Can you work these out from the model? Positions are in its coordinate system, mm. Face numbers are marked on the shaded views. A direction names the side the tool comes from. Give positions to 0.01 mm unless a question says otherwise; leave off trailing zeros. Order: outer loops, then holes, each group sorted by start corner. A loop starts at its lowest first (then second) coordinate and runs counter-clockwise, first axis right, second up. Notation, with made-up numbers: (3, -34) - (50, -34) arc R18 ccw to (50, -25) - close; hole circle Ø1 at (67, 73). An arc over 180 degrees is marked (long way). Return JSON: item names as keys, results as strings.
```python
from build123d import *

# Parameters (mm, degrees)
F1_DEPTH = 63.5
F0_W     = 25.4
F0_H     = 17.965186498
F2_DEPTH = 25.4
F3_DEPTH = 7.9375
F5_R     = 6.35


with BuildPart() as f1:
    # F0 (on Front) → F1 (new body, symmetric)
    with BuildSketch(Plane.XZ):
        Polygon((38.8800390695, 20.1806084275), (-24.6199609305, 20.1806084275), (-24.6199609305, 1.1306084275), (57.9300390695, 1.1306084275), (57.9300390695, 20.1806084275), align=None)
    extrude(amount=F1_DEPTH, both=True)

    # F0 (on Front) → F2 (join, symmetric)
    with BuildSketch(Plane.XZ):
        with Locations((91.4859331562, 62.5134016765)):
            Rectangle(F0_W, F0_H)
        with BuildLine():
            Line((38.8800390695, 36.0163077712), (38.8800390695, 20.1806084275))
            Line((38.8800390695, 20.1806084275), (57.9300390695, 20.1806084275))
            Line((57.9300390695, 20.1806084275), (57.9300390695, 36.5266351785))
            ThreePointArc((57.9300390695, 36.5266351785), (62.4384600836, 48.0819539272), (73.5812261701, 53.5308084275))
            Line((73.5812261701, 53.5308084275), (78.7859331562, 53.5308084275))
            Line((78.7859331562, 53.5308084275), (78.7859331562, 71.4959949255))
            Line((78.7859331562, 71.4959949255), (73.5812261701, 71.4959949255))
            add(Edge.make_bspline(
                [(73.0621663059, 71.4806777175), (73.2353354158, 71.485987393), (73.4083566499, 71.4910929714), (73.5812261701, 71.4959949255)],
                knots=[110.3659801148, 110.3659801148, 110.3659801148, 110.3659801148, 110.8004604656, 110.8004604656, 110.8004604656, 110.8004604656], degree=3))
            ThreePointArc((73.0621663059, 71.4806777175), (48.816685952, 60.6442358108), (38.8800390695, 36.0163077712))
        make_face()
    extrude(amount=F2_DEPTH, both=True)

    # F0 (on Front) → F3 (join, symmetric)
    with BuildSketch(Plane.XZ):
        with BuildLine():
            add(Edge.make_bspline(
                [(-24.6199609305, 20.1806084275), (-24.4558339647, 55.6137443141), (29.0740353989, 70.1319227371), (73.0621663059, 71.4806777175)],
                knots=[0, 0, 0, 0, 110.3659801148, 110.3659801148, 110.3659801148, 110.3659801148], degree=3))
            Line((-24.6199609305, 20.1806084275), (38.8800390695, 20.1806084275))
            Line((38.8800390695, 20.1806084275), (38.8800390695, 36.0163077712))
            ThreePointArc((38.8800390695, 36.0163077712), (48.816685952, 60.6442358108), (73.0621663059, 71.4806777175))
        make_face()
    extrude(amount=F3_DEPTH, both=True)

    # F0 (on Front) → F4 (revolve)
    with BuildSketch(Plane.XZ):
        Polygon((104.1859331562, 77.3306084275), (104.1859331562, 71.4959949255), (104.1859331562, 53.5308084275), (104.1859331562, 48.7556084275), (129.5859331562, 48.7556084275), (129.5859331562, 77.3306084275), align=None)
    revolve(axis=Axis((104.1859331562, 0, 63.0431084275), (0, 0, -1)))

    # F5
    f5_edges = [f1.edges().sort_by_distance(p)[0] for p in [
        (57.930039, 63.5, 10.655608),
        (57.930039, -63.5, 10.655608),
        (-24.619961, 63.5, 10.655608),
        (-24.619961, -63.5, 10.655608),
    ]]
    fillet(f5_edges, radius=F5_R)


solid = f1.part
```
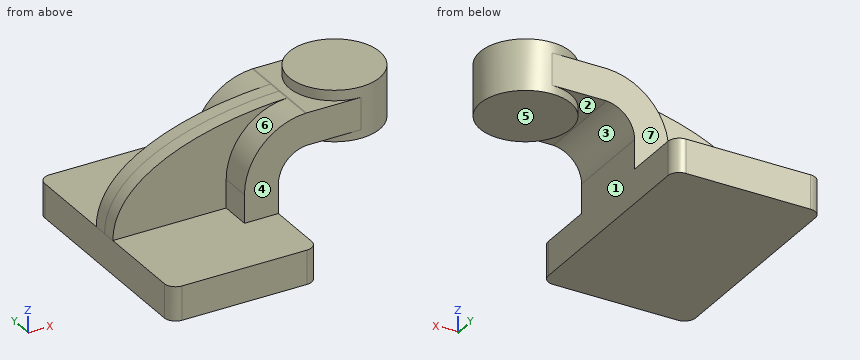
1. Thinking about a two-plate mould opening in X: for the marked faces 1, 2, 3 and 4, which applies, +X half, -X half, draft (parallel to the pull), parting line (faces both ways), or undercut?
Checks:
{"face 1": "+X half", "face 2": "undercut", "face 3": "undercut", "face 4": "draft"}
2. On a 3-axis mill with a long thin cutter (end or side, diameter ignored), from which of +Z, -Z, +X, -X, +Y, -Y can I reach the whole of each face in a straight line? I mean the marked faces 5, 6 and 7. Say none if no direction works.
Checks:
{"face 5": "-Z, +X, +Y, -Y", "face 6": "+Z, -X, -Y", "face 7": "+Z, +X, -X, +Y"}
3. If I drill on L1, parallel to Z at x = 32, y = 48; L2, parallel to Z at x = 86, y = -21; L3, parallel to X at y = -52.5, z = 8, over which ranges is the centre line in solid material (lowest first)? Write a range as [from, to].
Checks:
{"L1": "[1.13, 20.18]", "L2": "[53.53, 71.5]", "L3": "[-24.62, 57.93]"}
4. Suppose I cut it at B-B (y = -44). List the corners of the cut face in (x, z) for me.
Checks:
{"outline": "(-24.62, 1.13) - (57.93, 1.13) - (57.93, 20.18) - (-24.62, 20.18) - close"}
5. For pin 1 Ø16.5 at (x, y) = (5.5, -24) entering from +Z; pin 2 Ø5 at (x, z) = (50.5, 49.5) entering from +Y; pin 3 Ø2 at (y, z) = (23, 51) entering from +X, each with a flat end and sliding along its axis, tell me the tip position at first contact or that it passes through.
Checks:
{"pin 1": "z = 20.18", "pin 2": "y = 25.4", "pin 3": "x = 116.88"}
6. Suppose I cut it at A-A (z = 7). List the corners of the cut face in (x, y) for me, plus the area to 3 significant figures.
Checks:
{"outline": "(-24.62, -57.15) arc R6.35 ccw to (-18.27, -63.5) - (51.58, -63.5) arc R6.35 ccw to (57.93, -57.15) - (57.93, 57.15) arc R6.35 ccw to (51.58, 63.5) - (-18.27, 63.5) arc R6.35 ccw to (-24.62, 57.15) - close", "area": "10,400 mm^2"}
